Could you check a few things on this model? Use its own coordinates, in mm. Face numbers are marked on the shaded views. A direction names the side the tool comes from. Give positions to 0.01 mm unless a question says otherwise; leave off trailing zeros. Loops run counter-clockwise (first coordinate to the right, second up) from the corner with the lowest first, then second, coordinate; pieces in that order, holes last.
1. Imagine slicing it at B-B (x = -20.5). List the corners of the cut face in (y, z) for me.
2. Imagine slicing it at D-D (y = -11). List the corners of the cut face in (x, z) for me.
3. I need wall thicknesses on line 1 along X through (y, z) = (38, 3); line 2 along Y through (x, z) = (-8.5, 7); line 3 along Z through (x, y) = (-33, 43). Which ranges of each line are inside material? Lowest first, please.
4. Imagine slicing it at A-A (z = 5.25). List the corners of the cut face in (x, y) for me.
5. For P1, Ø5, axis at x = 93, z = 4, coming from the +Y side; P2, Ø3.5, axis at y = -2, z = 5, coming from the -X side; P3, Ø12, axis at x = 26.5, y = 18, coming from the -Z side, each with a flat end and sliding along its axis, tell me the tip position at first contact or that it passes through.
6. Thinking about a two-plate mould opening in X: for the marked faces 1 and 2, which applies, +X half, -X half, draft (parallel to the pull), parting line (faces both ways), or undercut?
7. For the marked faces 3, 4, 5, 6 and 7, which set-ups out of +Z, -Z, +X, -X, +Y, -Y let a thin tool reach every point of the face, with its end or its side?
8. Imagine slicing it at C-C (y = 23). List the corners of the cut face in (x, z) for me, plus the area to 3 significant figures.
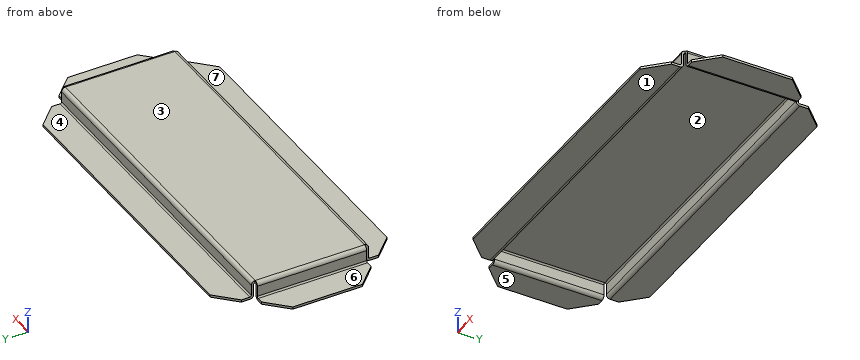
```python
from build123d import *

# Parameters (mm, degrees)
BASE_FLANGE1_DEPTH           = 55
EDGE_FLANGE1_DEPTH           = 168.5268
EDGE_FLANGE2_STRIP_W         = 6.2732
EDGE_FLANGE2_STRIP_H         = 1.2
EDGE_FLANGE2_STRIP_CUT_DEPTH = 168.5268
EDGE_FLANGE2_DEPTH           = 168.5268
EDGE_FLANGE3_DEPTH           = 168.5268
EDGE_FLANGE4_STRIP_W         = 6.2732
EDGE_FLANGE4_STRIP_H         = 1.2
EDGE_FLANGE4_STRIP_CUT_DEPTH = 168.5268
EDGE_FLANGE4_DEPTH           = 168.5268
CHAMFER1_SIZE                = 10


# Sheet-metal steps are written as plain solids
with BuildPart() as part:
    # Sketch1 → Base-Flange1 (new body)
    with BuildSketch(Plane(origin=(0, 0, 0), x_dir=(1, 0, 0), z_dir=(0, 1, 0))):
        with BuildLine():
            Line((-76.471389646, 0), (-63.407989646, 0))
            ThreePointArc((-63.407989646, 0), (-62.038606653, -0.567217008), (-61.471389646, -1.9366))
            Line((-61.471389646, -1.9366), (-61.471389646, -7.2634))
            ThreePointArc((-61.471389646, -7.2634), (-61.255644501, -7.784254855), (-60.734789646, -8))
            Line((-60.734789646, -8), (107.792010354, -8))
            ThreePointArc((107.792010354, -8), (108.312865209, -7.784254855), (108.528610354, -7.2634))
            Line((108.528610354, -7.2634), (108.528610354, -1.9366))
            ThreePointArc((108.528610354, -1.9366), (109.095827362, -0.567217008), (110.465210354, 0))
            Line((110.465210354, 0), (123.528610354, 0))
            Line((123.528610354, 0), (123.528610354, -1.2))
            Line((123.528610354, -1.2), (110.465210354, -1.2))
            ThreePointArc((110.465210354, -1.2), (109.944355499, -1.415745145), (109.728610354, -1.9366))
            Line((109.728610354, -1.9366), (109.728610354, -7.2634))
            ThreePointArc((109.728610354, -7.2634), (109.161393347, -8.632782992), (107.792010354, -9.2))
            Line((107.792010354, -9.2), (-60.734789646, -9.2))
            ThreePointArc((-60.734789646, -9.2), (-62.104172638, -8.632782992), (-62.671389646, -7.2634))
            Line((-62.671389646, -7.2634), (-62.671389646, -1.9366))
            ThreePointArc((-62.671389646, -1.9366), (-62.887134791, -1.415745145), (-63.407989646, -1.2))
            Line((-63.407989646, -1.2), (-76.471389646, -1.2))
            Line((-76.471389646, -1.2), (-76.471389646, 0))
        make_face()
    extrude(amount=BASE_FLANGE1_DEPTH)

    # Edge-Flange1 section (across the edge) → Edge-Flange1 (add)
    with BuildSketch(Plane(origin=(-60.734789646, 55.7366, 8), x_dir=(0, -1, 0), z_dir=(1, 0, 0))):
        with BuildLine():
            Line((-1.2, 0.7366), (-1.2, 8))
            Line((-1.2, 8), (0, 8))
            Line((0, 8), (0, 0.7366))
            ThreePointArc((0, 0.7366), (0.215745145, 0.215745145), (0.7366, 0))
            Line((0.7366, 0), (0.7366, -1.2))
            ThreePointArc((0.7366, -1.2), (-0.632782992, -0.632782992), (-1.2, 0.7366))
        make_face()
    extrude(amount=EDGE_FLANGE1_DEPTH)

    # Edge-Flange2 strip (across the edge) → Edge-Flange2 strip cut (cut)
    with BuildSketch(Plane(origin=(107.792010354, 56.9366, 0), x_dir=(0, 0, 1), z_dir=(-1, 0, 0))):
        with Locations((-1.2, -0.6)):
            Rectangle(EDGE_FLANGE2_STRIP_W, EDGE_FLANGE2_STRIP_H)
    extrude(amount=EDGE_FLANGE2_STRIP_CUT_DEPTH, mode=Mode.SUBTRACT)

    # Edge-Flange2 section (across the edge) → Edge-Flange2 (add)
    with BuildSketch(Plane(origin=(107.792010354, 56.9366, 0), x_dir=(0, 0, 1), z_dir=(-1, 0, 0))):
        with BuildLine():
            Line((0, 0.7366), (0, 15))
            Line((0, 15), (1.2, 15))
            Line((1.2, 15), (1.2, 0.7366))
            ThreePointArc((1.2, 0.7366), (1.415745145, 0.215745145), (1.9366, 0))
            Line((1.9366, 0), (1.9366, -1.2))
            ThreePointArc((1.9366, -1.2), (0.567217008, -0.632782992), (0, 0.7366))
        make_face()
    extrude(amount=EDGE_FLANGE2_DEPTH)

    # Edge-Flange3 section (across the edge) → Edge-Flange3 (add)
    with BuildSketch(Plane(origin=(107.792010354, -0.7366, 8), x_dir=(0, 1, 0), z_dir=(-1, 0, 0))):
        with BuildLine():
            Line((-1.2, 0.7366), (-1.2, 8))
            Line((-1.2, 8), (0, 8))
            Line((0, 8), (0, 0.7366))
            ThreePointArc((0, 0.7366), (0.215745145, 0.215745145), (0.7366, 0))
            Line((0.7366, 0), (0.7366, -1.2))
            ThreePointArc((0.7366, -1.2), (-0.632782992, -0.632782992), (-1.2, 0.7366))
        make_face()
    extrude(amount=EDGE_FLANGE3_DEPTH)

    # Edge-Flange4 strip (across the edge) → Edge-Flange4 strip cut (cut)
    with BuildSketch(Plane(origin=(-60.734789646, -1.9366, 0), x_dir=(0, 0, 1), z_dir=(1, 0, 0))):
        with Locations((-1.2, -0.6)):
            Rectangle(EDGE_FLANGE4_STRIP_W, EDGE_FLANGE4_STRIP_H)
    extrude(amount=EDGE_FLANGE4_STRIP_CUT_DEPTH, mode=Mode.SUBTRACT)

    # Edge-Flange4 section (across the edge) → Edge-Flange4 (add)
    with BuildSketch(Plane(origin=(-60.734789646, -1.9366, 0), x_dir=(0, 0, 1), z_dir=(1, 0, 0))):
        with BuildLine():
            Line((0, 0.7366), (0, 15))
            Line((0, 15), (1.2, 15))
            Line((1.2, 15), (1.2, 0.7366))
            ThreePointArc((1.2, 0.7366), (1.415745145, 0.215745145), (1.9366, 0))
            Line((1.9366, 0), (1.9366, -1.2))
            ThreePointArc((1.9366, -1.2), (0.567217008, -0.632782992), (0, 0.7366))
        make_face()
    extrude(amount=EDGE_FLANGE4_DEPTH)

    # Chamfer1
    chamfer1_edges = [part.edges().sort_by_distance(p)[0] for p in [
        (107.792010354, 71.9366, 0.6),
        (-60.734789646, 71.9366, 0.6),
        (-60.734789646, -16.9366, 0.6),
        (107.792010354, -16.9366, 0.6),
        (-76.471389646, 0, 0.6),
        (123.528610354, 0, 0.6),
        (-76.471389646, 55, 0.6),
        (123.528610354, 55, 0.6),
    ]]
    chamfer(chamfer1_edges, length=CHAMFER1_SIZE)


solid = part.part
```
Derived:
1. outline: (-16.94, 0) - (-2.67, 0) arc R1.94 ccw to (-0.74, 1.94) - (-0.74, 7.26) arc R0.74 cw to (0, 8) - (55, 8) arc R0.74 cw to (55.74, 7.26) - (55.74, 1.94) arc R1.94 ccw to (57.67, 0) - (71.94, 0) - (71.94, 1.2) - (57.67, 1.2) arc R0.74 cw to (56.94, 1.94) - (56.94, 7.26) arc R1.94 ccw to (55, 9.2) - (0, 9.2) arc R1.94 ccw to (-1.94, 7.26) - (-1.94, 1.94) arc R0.74 cw to (-2.67, 1.2) - (-16.94, 1.2) - close
2. outline: (-56.67, 0) - (103.73, 0) - (103.73, 1.2) - (-56.67, 1.2) - close
3. line 1: x = -62.67 to -61.47, 108.53 to 109.73
3. line 2: y = -1.94 to -0.74, 55.74 to 56.94
3. line 3: z = 8 to 9.2
4. outline: (-62.67, 0) - (-61.47, 0) - (-61.47, 55) - (-62.67, 55) - close; (-60.73, -1.94) - (107.79, -1.94) - (107.79, -0.74) - (-60.73, -0.74) - close; (-60.73, 55.74) - (107.79, 55.74) - (107.79, 56.94) - (-60.73, 56.94) - close; (108.53, 0) - (109.73, 0) - (109.73, 55) - (108.53, 55) - close
5. P1: stops at y = 57.08
5. P2: stops at x = -60.73
5. P3: stops at z = 8
6. face 1: draft
6. face 2: undercut
7. face 3: +Z, +X, -X, +Y, -Y
7. face 4: +Z, +X, -X, +Y
7. face 5: -Z, +X, -X, +Y, -Y
7. face 6: +Z, -X, +Y, -Y
7. face 7: +Z, +X, -X, -Y
8. outline: (-76.47, 0) - (-63.41, 0) arc R1.94 ccw to (-61.47, 1.94) - (-61.47, 7.26) arc R0.74 cw to (-60.73, 8) - (107.79, 8) arc R0.74 cw to (108.53, 7.26) - (108.53, 1.94) arc R1.94 ccw to (110.47, 0) - (123.53, 0) - (123.53, 1.2) - (110.47, 1.2) arc R0.74 cw to (109.73, 1.94) - (109.73, 7.26) arc R1.94 ccw to (107.79, 9.2) - (-60.73, 9.2) arc R1.94 ccw to (-62.67, 7.26) - (-62.67, 1.94) arc R0.74 cw to (-63.41, 1.2) - (-76.47, 1.2) - close
8. area: 256 mm2
